Check sheet for the modelled part. Datum: model origin and axes. Units: mm. Face numbers are marked on the shaded views. Coordinates: 2 decimals unless noted, no trailing zeros. Order: outer loops, then holes, each group sorted by start corner. A loop starts at its lowest first (then second) coordinate and runs counter-clockwise, first axis right, second up. Notation, with made-up numbers: (65, 82) -> (110, 82) arc R16 ccw to (110, 101) -> close; hole circle Ø3 at (-13, -10.5). An arc over 180 degrees is marked (long way). Put each result on its own line as item: value. Start each with the question number.
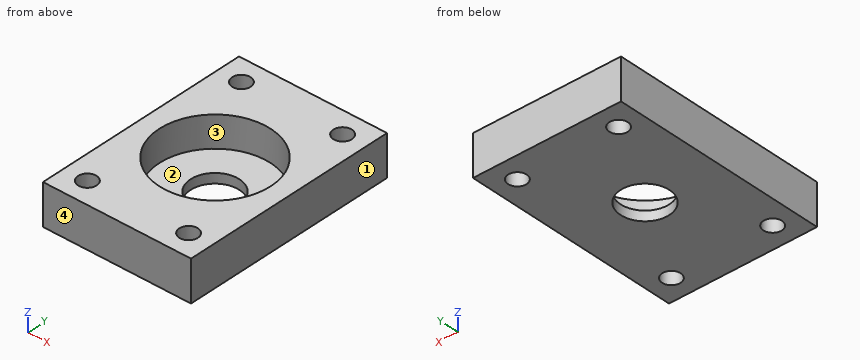
```python
from build123d import *

# Parameters (mm, degrees)
CROQUIS1_R              = 18.2875
CROQUIS1_R_2            = 14.2875
SALIENTE_EXTRUIR1_DEPTH = 8
CROQUIS2_W              = 38
CROQUIS2_H              = 56
CROQUIS2_R              = 18.2875
SALIENTE_EXTRUIR2_DEPTH = 8
CROQUIS5_W              = 38
CROQUIS5_H              = 56
CROQUIS5_R              = 6.25
SALIENTE_EXTRUIR3_DEPTH = 2.5
CROQUIS7_R              = 2.38125
CORTAR_EXTRUIR3_DEPTH   = 11.5


with BuildPart() as part:
    # Croquis1 → Saliente-Extruir1 (new body)
    with BuildSketch(Plane.XY):
        Circle(CROQUIS1_R)
        Circle(CROQUIS1_R_2, mode=Mode.SUBTRACT)
    extrude(amount=SALIENTE_EXTRUIR1_DEPTH)

    # Croquis2 → Saliente-Extruir2 (add)
    with BuildSketch(Plane(origin=(0, 0, 0), x_dir=(-1, 0, 0), z_dir=(0, 0, -1))):
        Rectangle(CROQUIS2_W, CROQUIS2_H)
        Circle(CROQUIS2_R, mode=Mode.SUBTRACT)
    extrude(amount=-SALIENTE_EXTRUIR2_DEPTH)

    # Croquis5 → Saliente-Extruir3 (add)
    with BuildSketch(Plane(origin=(0, 0, 0), x_dir=(-1, 0, 0), z_dir=(0, 0, -1))):
        Rectangle(CROQUIS5_W, CROQUIS5_H)
        Circle(CROQUIS5_R, mode=Mode.SUBTRACT)
    extrude(amount=SALIENTE_EXTRUIR3_DEPTH)

    # Croquis7 → Cortar-Extruir3 (cut, through all)
    with BuildSketch(Plane(origin=(0, 0, -2.5), x_dir=(-1, 0, 0), z_dir=(0, 0, -1))):
        with Locations((-13, 22)):
            Circle(CROQUIS7_R)
        with Locations((13, 22)):
            Circle(CROQUIS7_R)
        with Locations((13, -22)):
            Circle(CROQUIS7_R)
        with Locations((-13, -22)):
            Circle(CROQUIS7_R)
    extrude(amount=-CORTAR_EXTRUIR3_DEPTH, mode=Mode.SUBTRACT)


solid = part.part
```
1) Sectioned sample at B-B (y = 0). Record the boundary of the cut face in (x, z), plus the area to 3 significant figures.
2) Scan lines: line 1 along Y through (x, z) = (13, 3); line 2 along X through (y, z) = (-20, 2.5); line 3 along X through (y, z) = (21, 5.75). Record each from-to range of solid material in increasing order. Write a range as [from, to].
3) Sectioned sample at C-C (y = -22). Record the boundary of the cut face in (x, z), plus the area to 3 significant figures.
4) Sectioned sample at A-A (x = 0). Record the boundary of the cut face in (y, z).
5) Gauge pin test, flat end, axial feed: pin 1 (8.5 mm diameter, centred on x = 5, y = 0.5, fed in from +Z). Record the tip position at first contact, or that the pin passes through.
6) Mould release check, pull along X, two halves, no side actions. Record for the marked faces 1, 2, 3 and 4: +X half, -X half, draft (parallel to the pull), parting line (faces both ways), or undercut.
7) Sectioned sample at D-D (z = 2.25). Record the boundary of the cut face in (x, y) (1 decimal), plus the area to 3 significant figures.
Entries:
1. outline: (-19, -2.5) -> (-6.25, -2.5) -> (-6.25, 0) -> (-14.29, 0) -> (-14.29, 8) -> (-19, 8) -> close; (6.25, -2.5) -> (19, -2.5) -> (19, 8) -> (14.29, 8) -> (14.29, 0) -> (6.25, 0) -> close
1. area: 139 mm2
2. line 1: y = [-28, -24.38], [-19.62, -5.93], [5.93, 19.62], [24.38, 28]
2. line 2: x = [-19, -14.29], [-11.71, 11.71], [14.29, 19]
2. line 3: x = [-19, -15.16], [-10.84, 10.84], [15.16, 19]
3. outline: (-19, -2.5) -> (-15.38, -2.5) -> (-15.38, 8) -> (-19, 8) -> close; (-10.62, -2.5) -> (10.62, -2.5) -> (10.62, 8) -> (-10.62, 8) -> close; (15.38, -2.5) -> (19, -2.5) -> (19, 8) -> (15.38, 8) -> close
3. area: 299 mm2
4. outline: (-28, -2.5) -> (-6.25, -2.5) -> (-6.25, 0) -> (-14.29, 0) -> (-14.29, 8) -> (-28, 8) -> close; (6.25, -2.5) -> (28, -2.5) -> (28, 8) -> (14.29, 8) -> (14.29, 0) -> (6.25, 0) -> close
5. pin 1: stops at z = 0
6. face 1: +X half
6. face 2: undercut
6. face 3: undercut
6. face 4: draft
7. outline: (-19, -28) -> (19, -28) -> (19, 28) -> (-19, 28) -> close; hole circle Ø4.8 at (-13, -22); hole circle Ø4.8 at (-13, 22); hole circle Ø28.6 at (0, 0); hole circle Ø4.8 at (13, -22); hole circle Ø4.8 at (13, 22)
7. area: 1,420 mm2
